Build history of the part. All positions in model axes, mm. A direction names the side the tool comes from. Round coordinates to 2 decimals unless told otherwise and drop trailing zeros. Order: outer loops, then holes, each group sorted by start corner. A loop starts at its lowest first (then second) coordinate and runs counter-clockwise, first axis right, second up. Notation, with made-up numbers: (86.5, 17.25) -> (143.5, 17.25) arc R10 ccw to (143.5, 36.25) -> close; hole circle Ø9 at (55, -20). An arc over 180 degrees is marked (long way). Write item = value, one per line.
from build123d import *

# Parameters (mm, degrees)
SKETCH_1_R          = 2.75
EXTRUDE_1_DEPTH     = 9
SKETCH_3_W          = 42
SKETCH_3_H          = 42
SKETCH_3_R          = 1.75
SKETCH_3_R_2        = 12
EXTRUDE_2_DEPTH     = 6
SKETCH_4_R          = 3
CUT_EXTRUDE_2_DEPTH = 3
SKETCH_5_W          = 42
SKETCH_5_H          = 9
EXTRUDE_3_DEPTH     = 6
SKETCH_6_R          = 4.25
CUT_EXTRUDE_3_DEPTH = 5
CHAMFER_2_SIZE      = 5
SKETCH_7_W          = 51
SKETCH_7_H          = 6
EXTRUDE_4_DEPTH     = 9
CHAMFER_3_SIZE      = 5
FILLET_1_R          = 0.5


with BuildPart() as part:
    # Sketch 1 → Extrude 1 (new body)
    with BuildSketch(Plane.XY):
        Polygon((30, 21), (21, 21), (-21, 21), (-21, -21), (21, -21), (30, -21), align=None)
        with Locations((0, 15)):
            Circle(SKETCH_1_R, mode=Mode.SUBTRACT)
        with Locations((20, 15)):
            Circle(SKETCH_1_R, mode=Mode.SUBTRACT)
        with Locations((20, 0)):
            Circle(SKETCH_1_R, mode=Mode.SUBTRACT)
        with Locations((20, -15)):
            Circle(SKETCH_1_R, mode=Mode.SUBTRACT)
        Circle(SKETCH_1_R, mode=Mode.SUBTRACT)
        with Locations((0, -15)):
            Circle(SKETCH_1_R, mode=Mode.SUBTRACT)
    extrude(amount=EXTRUDE_1_DEPTH)



with BuildPart() as body_2:
    # Sketch 3 → Extrude 2 (new body)
    with BuildSketch(Plane.XZ.offset(21)):
        with Locations((0, 30)):
            Rectangle(SKETCH_3_W, SKETCH_3_H)
        with Locations(Location((-15.5, 45.5, 0), (0, 0, 270))):
            Circle(SKETCH_3_R, mode=Mode.SUBTRACT)
        with Locations(Location((-15.5, 14.5, 0), (0, 0, 90))):
            Circle(SKETCH_3_R, mode=Mode.SUBTRACT)
        with Locations(Location((15.5, 14.5, 0), (0, 0, 270))):
            Circle(SKETCH_3_R, mode=Mode.SUBTRACT)
        with Locations(Location((15.5, 45.5, 0), (0, 0, 90))):
            Circle(SKETCH_3_R, mode=Mode.SUBTRACT)
        with Locations(Location((0, 30, 0), (0, 0, 270))):
            Circle(SKETCH_3_R_2, mode=Mode.SUBTRACT)
    extrude(amount=EXTRUDE_2_DEPTH)

    # Sketch 4 → Cut-Extrude 2 (cut)
    with BuildSketch(Plane.XZ.offset(27)):
        with Locations(Location((-15.5, 45.5, 0), (0, 0, 270))):
            Circle(SKETCH_4_R)
        with Locations(Location((-15.5, 14.5, 0), (0, 0, 90))):
            Circle(SKETCH_4_R)
        with Locations(Location((15.5, 14.5, 0), (0, 0, 270))):
            Circle(SKETCH_4_R)
        with Locations(Location((15.5, 45.5, 0), (0, 0, 90))):
            Circle(SKETCH_4_R)
    extrude(amount=-CUT_EXTRUDE_2_DEPTH, mode=Mode.SUBTRACT)


with BuildPart() as part_1:
    add(part.part)

    add(body_2.part)  # Extrude 3 merges body 2
    # Sketch 5 → Extrude 3 (add)
    with BuildSketch(Plane.XZ.offset(21)):
        with Locations((0, 4.5)):
            Rectangle(SKETCH_5_W, SKETCH_5_H)
    extrude(amount=EXTRUDE_3_DEPTH)

    # Sketch 6 → Cut-Extrude 3 (cut)
    with BuildSketch(Plane.XY.offset(9)):
        with Locations((0, 15)):
            Circle(SKETCH_6_R)
        with Locations((20, 15)):
            Circle(SKETCH_6_R)
        with Locations((20, 0)):
            Circle(SKETCH_6_R)
        with Locations((20, -15)):
            Circle(SKETCH_6_R)
        Circle(SKETCH_6_R)
        with Locations((0, -15)):
            Circle(SKETCH_6_R)
    extrude(amount=-CUT_EXTRUDE_3_DEPTH, mode=Mode.SUBTRACT)

    # Chamfer 2
    chamfer_2_edges = [part_1.edges().sort_by_distance(p)[0] for p in [
        (-21, 21, 4.5),
        (30, 21, 4.5),
    ]]
    chamfer(chamfer_2_edges, length=CHAMFER_2_SIZE)

    # Sketch 7 → Extrude 4 (add)
    with BuildSketch(Plane(origin=(21, 0, 0), x_dir=(0, 0, -1), z_dir=(1, 0, 0))):
        with Locations((-25.5, -24)):
            Rectangle(SKETCH_7_W, SKETCH_7_H)
    extrude(amount=EXTRUDE_4_DEPTH)

    # Chamfer 3
    chamfer_3_edges = [part_1.edges().sort_by_distance(p)[0] for p in [
        (30, -24, 51),
        (-21, -24, 51),
    ]]
    chamfer(chamfer_3_edges, length=CHAMFER_3_SIZE)

    # Fillet 1
    fillet_1_edges = [part_1.edges().sort_by_distance(p)[0] for p in [
        (4.5, -21, 9),
    ]]
    fillet(fillet_1_edges, radius=FILLET_1_R)


solid = part_1.part
Q1. Flat gauge pins, fed straight in: pin 1 (7 mm diameter, centred on x = 0, y = -15, fed in from +Z); pin 2 (11 mm diameter, centred on x = 20, y = -15, fed in from +Z); pin 3 (1.5 mm diameter, centred on x = 20.5, z = 32, fed in from +Y). Where does each tip first touch, or does it go through?
Check values:
pin_1 = 4
pin_2 = 9
pin_3 = -21
Q2. Cut at D-D, the plane x = 26. List the corners of the cut face in (y, z), and give its area (3 significant figures).
Check values:
outline = (-27, 0) -> (20, 0) -> (20, 9) -> (-20.5, 9) arc R0.5 cw to (-21, 9.5) -> (-21, 50) -> (-27, 50) -> close
area = 669 mm²
Q3. Mould opens along Y. For faces 5 (the face through (-14.974, -22.479, 43.831)), 6 (the face through (-0.596, -2.685, 1.972)), 7 (the face through (10, -21, 21)) say: released by +Y, released by -Y, zero draft, split by the parting line, or undercut.
Check values:
face_5 = zero draft
face_6 = undercut
face_7 = released by +Y
Q4. Cut at A-A, the plane y = 15. List the corners of the cut face in (x, z), and give its area (3 significant figures).
Check values:
outline = (-21, 0) -> (-2.75, 0) -> (-2.75, 4) -> (-4.25, 4) -> (-4.25, 9) -> (-21, 9) -> close; (2.75, 0) -> (17.25, 0) -> (17.25, 4) -> (15.75, 4) -> (15.75, 9) -> (4.25, 9) -> (4.25, 4) -> (2.75, 4) -> close; (22.75, 0) -> (30, 0) -> (30, 9) -> (24.25, 9) -> (24.25, 4) -> (22.75, 4) -> close
area = 330 mm²
Q5. Probe probe 1 along Z at (x, y) = (-15.5, -23.1); probe 2 along X at (y, z) = (-24.9, 14.5); probe 3 along Y at (x, z) = (0, 6). List the from-to ranges inside material, lowest first.
Check values:
probe_1 = 0 to 12.75, 16.25 to 43.75, 47.25 to 51
probe_2 = -21 to -18.5, -12.5 to 12.5, 18.5 to 30
probe_3 = -27 to -19.25, -10.75 to -4.25, 4.25 to 10.75, 19.25 to 21
Q6. Cut at B-B, the plane z = 30. List the corners of the cut face in (x, y).
Check values:
outline = (-21, -27) -> (-12, -27) -> (-12, -21) -> (-21, -21) -> close; (12, -27) -> (30, -27) -> (30, -21) -> (12, -21) -> close
Q7. Cut at C-C, the plane x = 20. Give the number of separate pieces and of enclosed holes in the cut face, and give its area (3 significant figures).
Check values:
separate_pieces = 4
enclosed_holes = 0
area = 491 mm²
Q8. Which spindle directions (+Z, -Z, +X, -X, +Y, -Y) get a long thin tool onto all of the face, cutting with end or side? Do faces 1 (the face through (17.3, -25.5, 43.1)), 2 (the face through (17, -22.5, 13.6)), 3 (the face through (0, -18, 4)), 4 (the face through (4, -4, 9)). Say none if no direction does.
Check values:
face_1 = -Y
face_2 = +Y, -Y
face_3 = +Z
face_4 = +Z, +X, -X, +Y
